Source: CAD feature listing. Evaluate the final solid. Frame: model axes, mm. Face numbers are marked on the shaded views. A direction names the side the tool comes from. Coordinates: 2 decimals unless noted, no trailing zeros. Loops run counter-clockwise (first coordinate to the right, second up) from the corner with the lowest first, then second, coordinate; pieces in that order, holes last.
Item 1: Line query: probe 1 along Z at (x, y) = (37.5, 40.5); probe 2 along Y at (x, z) = (42, 59); probe 3 along Z at (x, y) = (30, -4). Output: solid intervals per line, ascending.
Item 2: Reachability of the marked faces 5 and 6 from +Z, -Z, +X, -X, +Y, -Y: full face, straight path, thin tool, end or side. Return the list, or none.
Item 3: Section query D-D, the plane z = 69.5. Return the cut outline in (x, y), then the cut area to 3 significant figures.
Item 4: Pull-direction query (Z, two-part tool) for the marked faces 1, 2, 3 and 4; classes: +Z half, -Z half, draft (parallel to the pull), parting line (faces both ways), or undercut.
Item 5: Section query B-B, the plane x = 56. Return the cut outline in (y, z).
Item 6: Pin query (flat end, axial travel): pin 1 Ø3 at (y, z) = (12, 9) entering from +X; pin 2 Ø4 at (x, z) = (30, 30.53) entering from -Y. Return the tip coordinate at first contact, or that it passes through.
Item 7: Section query C-C, the plane y = 29.5. Return the cut outline in (x, z), then the cut area to 3 significant figures.
Item 8: Section query A-A, the plane x = 30. Return the cut outline in (y, z).
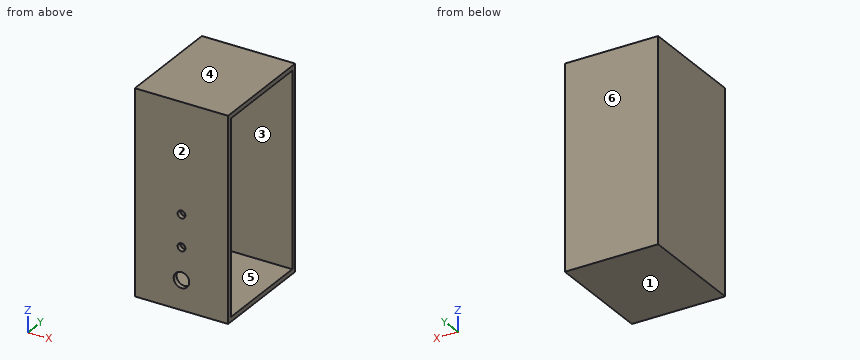
```python
from build123d import *

# Parameters (mm, degrees)
F0_W     = 70
F0_H     = 130
F1_DEPTH = 60
F2_T     = -3
F3_R     = 5
F3_R_2   = 2.5
F4_DEPTH = 3


with BuildPart() as f1:
    # F0 (on Right) → F1 (new body)
    with BuildSketch(Plane.YZ):
        with Locations((30.021758, 56.224507)):
            Rectangle(F0_W, F0_H)
    extrude(amount=F1_DEPTH)

    # F2
    f2_openings = [f1.faces().sort_by_distance(p)[0] for p in [
        (60, 30.021758, 56.224507),
    ]]
    offset(amount=F2_T, openings=f2_openings)

    # F3 (on face) → F4 (cut, through all)
    with BuildSketch(Plane.XZ.offset(4.978242)):
        with Locations((30, 10.026326)):
            Circle(F3_R)
        with Locations((30, 30.526326)):
            Circle(F3_R_2)
        with Locations((30, 51.026326)):
            Circle(F3_R_2)
    extrude(amount=-F4_DEPTH, mode=Mode.SUBTRACT)


solid = f1.part
```
Verdict:
1. probe 1: z = -8.78 to -5.78, 118.22 to 121.22
1. probe 2: y = -4.98 to -1.98, 62.02 to 65.02
1. probe 3: z = -8.78 to 5.03, 15.03 to 28.03, 33.03 to 48.53, 53.53 to 121.22
2. face 5: +X
2. face 6: +Z, -Z, +X, -X, +Y
3. outline: (0, -4.98) - (60, -4.98) - (60, -1.98) - (3, -1.98) - (3, 62.02) - (60, 62.02) - (60, 65.02) - (0, 65.02) - close
3. area: 552 mm2
4. face 1: -Z half
4. face 2: draft
4. face 3: undercut
4. face 4: +Z half
5. outline: (-4.98, -8.78) - (65.02, -8.78) - (65.02, 121.22) - (-4.98, 121.22) - close; hole (-1.98, -5.78) - (62.02, -5.78) - (62.02, 118.22) - (-1.98, 118.22) - close
6. pin 1: stops at x = 3
6. pin 2: stops at y = 62.02
7. outline: (0, -8.78) - (60, -8.78) - (60, -5.78) - (3, -5.78) - (3, 118.22) - (60, 118.22) - (60, 121.22) - (0, 121.22) - close
7. area: 732 mm2
8. outline: (-4.98, -8.78) - (65.02, -8.78) - (65.02, 121.22) - (-4.98, 121.22) - (-4.98, 53.53) - (-1.98, 53.53) - (-1.98, 118.22) - (62.02, 118.22) - (62.02, -5.78) - (-1.98, -5.78) - (-1.98, 5.03) - (-4.98, 5.03) - close; (-4.98, 15.03) - (-1.98, 15.03) - (-1.98, 28.03) - (-4.98, 28.03) - close; (-4.98, 33.03) - (-1.98, 33.03) - (-1.98, 48.53) - (-4.98, 48.53) - close
